Here's how the part is built. I have some questions about the finished solid (model axes, mm). Face numbers are marked on the shaded views. A direction names the side the tool comes from. Give positions to 0.01 mm unless a question says otherwise; leave off trailing zeros. Loops run counter-clockwise (first coordinate to the right, second up) from the corner with the lowest first, then second, coordinate; pieces in that order, holes last. Notation, with made-up numbers: (65.25, 1) -> (90.25, 1) arc R28 ccw to (90.25, 34) -> close; hole circle Ø1 at (32, -24). An arc over 180 degrees is marked (long way). Answer in a Markdown table with one row per item. Add a question column.
Item 1: If I drill on line 1 (Y direction, x = 19, z = -6); line 2 (X direction, y = 45, z = -6.25); line 3 (Z direction, x = 41.5, y = 33), over which ranges is the centre line in solid material (lowest first)?
Item 2: If we section it at C-C (x = 41.5): Write out the boundary of the cut face in (y, z).
Item 3: We'd pull the mould along X, two halves only. Please class the marked faces 1, 2 and 3: released by +X, released by -X, zero draft, split by the parting line, or undercut.
Item 4: If we section it at B-B (y = 34): Write out the boundary of the cut face in (x, z).
Item 5: If we section it at A-A (y = 60): Write out the boundary of the cut face in (x, z), then the cut area to 3 significant figures.
Item 6: Which directions (+Z, -Z, +X, -X, +Y, -Y) give clear straight access to the entire face, cutting with the end or side of a thin tool? Please do the marked faces 4, 5 and 6.
Item 7: For P1, Ø6.5, axis at x = 41.5, z = -6, coming from the +Y side; P2, Ø3, axis at y = 57.5, z = -8, coming from the +X side; P3, Ø4, axis at x = 46.5, z = -3.5, coming from the -Y side; P4, Ø6, axis at x = 43, y = 49.5, coming from the +Z side, each with a flat end and sliding along its axis, tell me the tip position at first contact or that it passes through.
Item 8: If we section it at D-D (z = -6): Give the number of separate pieces and of enclosed holes in the cut face, then the cut area to 3 significant figures.
```python
from build123d import *

# Parameters (mm, degrees)
BOSS_EXTRUDE1_DEPTH      = 12
SKETCH2_R                = 2.1
CUT_EXTRUDE1_DEPTH       = 82.983229992
M5_CLEARANCE_HOLE1_D     = 5.5
M5_CLEARANCE_HOLE1_DEPTH = 28.347633298
M5_CLEARANCE_HOLE1_TIP   = 1.652366702
FILLET1_R                = 2.55
CHAMFER1_SIZE            = 1


with BuildPart() as part:
    # Sketch1 → Boss-Extrude1 (new body)
    with BuildSketch(Plane.XY):
        Polygon((10, 65), (10, 8), (33.5, 8), (33.5, 22.7), (58.5, 22.7), (58.5, 50.3), (33.5, 50.3), (33.5, 65), align=None)
    extrude(amount=-BOSS_EXTRUDE1_DEPTH)

    # Sketch2 → Cut-Extrude1 (cut, through all)
    with BuildSketch(Plane.ZY.offset(-10)):
        with Locations((-6, 13)):
            Circle(SKETCH2_R)
        with Locations((-6, 60)):
            Circle(SKETCH2_R)
    extrude(amount=-CUT_EXTRUDE1_DEPTH, mode=Mode.SUBTRACT)

    # M5 Clearance Hole1
    with Locations(Plane(origin=(0, 22.7, 0), x_dir=(-1, 0, 0), z_dir=(0, -1, 0))):
        with Locations((-53.5, 6), (-41.5, 6)):
            Hole(M5_CLEARANCE_HOLE1_D / 2, depth=M5_CLEARANCE_HOLE1_DEPTH)
            with Locations((0, 0, -(M5_CLEARANCE_HOLE1_DEPTH + M5_CLEARANCE_HOLE1_TIP / 2))):  # 118° drill point
                Cone(0, M5_CLEARANCE_HOLE1_D / 2, M5_CLEARANCE_HOLE1_TIP, mode=Mode.SUBTRACT)

    # Fillet1
    # the kernel refuses this fillet: 2.55 mm, written as the material it adds along each edge
    with BuildSketch(Plane(origin=(33.5, 50.3, 0), x_dir=(0, 1, 0), z_dir=(0, 0, -1))) as fillet1_piece_1:
        with BuildLine():
            CenterArc((FILLET1_R, FILLET1_R), FILLET1_R, 180, 90)
            Line((0, FILLET1_R), (0, 0))
            Line((0, 0), (FILLET1_R, 0))
        make_face()
    extrude(amount=12)
    with BuildSketch(Plane(origin=(33.5, 22.7, 0), x_dir=(0, -1, 0), z_dir=(0, 0, -1))) as fillet1_piece_2:
        with BuildLine():
            CenterArc((FILLET1_R, -FILLET1_R), FILLET1_R, 90, 90)
            Line((0, -FILLET1_R), (0, 0))
            Line((0, 0), (FILLET1_R, 0))
        make_face()
    extrude(amount=12)
    # the kernel refuses this fillet: 2.55 mm, written as the material it takes off along each edge
    with BuildSketch(Plane(origin=(33.5, 65, 6.375), x_dir=(-1, 0, 0), z_dir=(0, 0, -1)), Plane(origin=(10, 65, 6.375), x_dir=(0, -1, 0), z_dir=(0, 0, -1))) as fillet1_2_piece_1:
        with BuildLine():
            CenterArc((FILLET1_R, -FILLET1_R), FILLET1_R, 90, 90)
            Line((0, -FILLET1_R), (0, 0))
            Line((0, 0), (FILLET1_R, 0))
        make_face()
    extrude(amount=24.75, mode=Mode.SUBTRACT)
    with BuildSketch(Plane(origin=(58.5, 50.3, 6.375), x_dir=(0, -1, 0), z_dir=(0, 0, -1)), Plane(origin=(58.5, 22.7, 6.375), x_dir=(-1, 0, 0), z_dir=(0, 0, -1)), Plane(origin=(33.5, 8, 6.375), x_dir=(-1, 0, 0), z_dir=(0, 0, -1)), Plane(origin=(10, 8, 6.375), x_dir=(0, 1, 0), z_dir=(0, 0, -1))) as fillet1_2_piece_2:
        with BuildLine():
            CenterArc((FILLET1_R, FILLET1_R), FILLET1_R, 180, 90)
            Line((0, FILLET1_R), (0, 0))
            Line((0, 0), (FILLET1_R, 0))
        make_face()
    extrude(amount=24.75, mode=Mode.SUBTRACT)

    # Chamfer1
    chamfer1_edges = [part.edges().sort_by_distance(p)[0] for p in [
        (58.5, 36.5, 0),
        (21.75, 65, 0),
        (10, 36.5, 0),
        (21.75, 8, 0),
        (33.5, 15.35, 0),
        (46, 22.7, 0),
        (46, 50.3, 0),
        (33.5, 57.65, 0),
        (57.753122292, 23.446877708, 0),
        (32.753122292, 8.746877708, 0),
        (10.746877708, 8.746877708, 0),
        (10.746877708, 64.253122292, 0),
        (32.753122292, 64.253122292, 0),
        (57.753122292, 49.553122292, 0),
        (34.246877708, 51.046877708, 0),
        (34.246877708, 21.953122292, 0),
    ]]
    chamfer(chamfer1_edges, length=CHAMFER1_SIZE)


solid = part.part
```
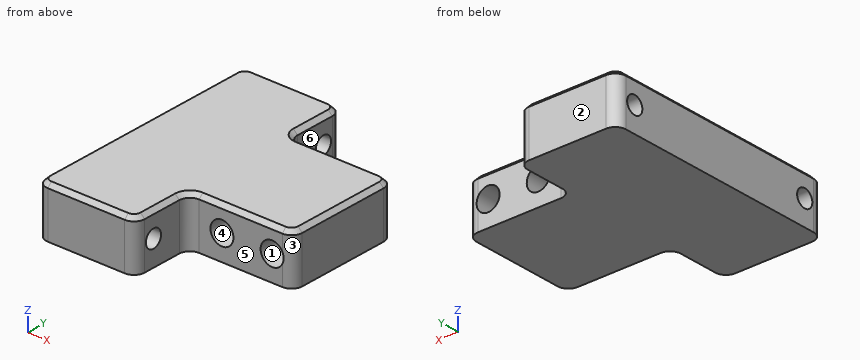
Recorded:
| question | item | result |
|---|---|---|
| 1 | line 1 | y = 8 to 10.9, 15.1 to 57.9, 62.1 to 65 |
| 1 | line 2 | x = 10 to 38.76, 44.24 to 50.76, 56.24 to 58.5 |
| 1 | line 3 | z = -12 to -8.75, -3.25 to 0 |
| 2 | outline | (22.7, -12) -> (50.3, -12) -> (50.3, -8.75) -> (22.7, -8.75) -> close; (22.7, -3.25) -> (50.3, -3.25) -> (50.3, -1) -> (49.3, 0) -> (23.7, 0) -> (22.7, -1) -> close |
| 3 | face 1 | undercut |
| 3 | face 2 | zero draft |
| 3 | face 3 | released by +X |
| 4 | outline | (10, -12) -> (58.5, -12) -> (58.5, -1) -> (57.5, 0) -> (11, 0) -> (10, -1) -> close; hole circle Ø5.5 at (41.5, -6); hole circle Ø5.5 at (53.5, -6) |
| 5 | outline | (10, -12) -> (33.5, -12) -> (33.5, -8.1) -> (10, -8.1) -> close; (10, -3.9) -> (33.5, -3.9) -> (33.5, -1) -> (32.5, 0) -> (11, 0) -> (10, -1) -> close |
| 5 | area | 182 mm^2 |
| 6 | face 4 | +Y, -Y |
| 6 | face 5 | +Z, -Z, +X, -Y |
| 6 | face 6 | +Z, -Z, +X, +Y |
| 7 | P1 | stops at y = 50.3 |
| 7 | P2 | stops at x = 33.5 |
| 7 | P3 | stops at y = 22.7 |
| 7 | P4 | stops at z = 0 |
| 8 | separate pieces | 5 |
| 8 | enclosed holes | 0 |
| 8 | area | 1,520 mm^2 |
